Autodesk Inventor part; units mm, degrees
ref_plane "Work Plane3" through (0, 0, 250) normal (0, 0, 1) x (1, 0, 0)
ref_plane "Start Plane" through (0, 0, 0) normal (0, 0, 1) x (1, 0, 0)
ref_plane "End Plane" through (0, 0, 450) normal (0, 0, 1) x (1, 0, 0)
sketch "Sketch" plane through (0, 0, 0) normal (0, 0, 1) x (1, 0, 0)
  line L0 (-13, 15) -> (13, 15)
  line L1 (15, 13) -> (15, -13)
  line L2 (-15, 15) -> (15, -15) construction
  line L3 (15, 15) -> (-15, -15) construction
  line L4 (-5.2, 15) -> (-5.2, 14.2)
  line L5 (-5.2, 14.2) -> (-4.1, 14.2)
  line L6 (-4.1, 14.2) -> (-4.1, 12.2)
  line L7 (-4.1, 12.2) -> (-8.25, 12.2)
  line L8 (-8.25, 12.2) -> (-8.25, 10.2)
  line L9 (-8.25, 10.2) -> (-3.85, 5.8)
  line L10 (-3.85, 5.8) -> (3.85, 5.8)
  line L11 (8.25, 12.2) -> (4.1, 12.2)
  line L12 (4.1, 12.2) -> (4.1, 14.2)
  line L13 (4.1, 14.2) -> (5.2, 14.2)
  line L14 (5.2, 14.2) -> (5.2, 15)
  line L15 (8.25, 12.2) -> (8.25, 10.2)
  line L16 (8.25, 10.2) -> (3.85, 5.8)
  line L17 (-2.5, 0) -> (0, 0)
  line L18 (-5.2, -15) -> (-5.2, -14.2)
  line L19 (-5.2, -14.2) -> (-4.1, -14.2)
  line L20 (-4.1, -14.2) -> (-4.1, -12.2)
  line L21 (-4.1, -12.2) -> (-8.25, -12.2)
  line L22 (-8.25, -12.2) -> (-8.25, -10.2)
  line L23 (-8.25, -10.2) -> (-3.85, -5.8)
  line L24 (-3.85, -5.8) -> (3.85, -5.8)
  line L25 (8.25, -12.2) -> (4.1, -12.2)
  line L26 (4.1, -12.2) -> (4.1, -14.2)
  line L27 (4.1, -14.2) -> (5.2, -14.2)
  line L28 (5.2, -14.2) -> (5.2, -15)
  line L29 (8.25, -12.2) -> (8.25, -10.2)
  line L30 (8.25, -10.2) -> (3.85, -5.8)
  line L31 (15, 5.2) -> (14.2, 5.2)
  line L32 (14.2, 5.2) -> (14.2, 4.1)
  line L33 (14.2, 4.1) -> (12.2, 4.1)
  line L34 (12.2, 4.1) -> (12.2, 8.25)
  line L35 (15, -5.2) -> (14.2, -5.2)
  line L36 (14.2, -5.2) -> (14.2, -4.1)
  line L37 (14.2, -4.1) -> (12.2, -4.1)
  line L38 (12.2, -4.1) -> (12.2, -8.25)
  line L39 (12.2, -8.25) -> (10.2, -8.25)
  line L40 (10.2, -8.25) -> (5.8, -3.85)
  line L41 (5.8, -3.85) -> (5.8, 3.85)
  line L42 (5.8, 3.85) -> (10.2, 8.25)
  line L43 (10.2, 8.25) -> (12.2, 8.25)
  line L44 (-15, 5.2) -> (-14.2, 5.2)
  line L45 (-14.2, 5.2) -> (-14.2, 4.1)
  line L46 (-14.2, 4.1) -> (-12.2, 4.1)
  line L47 (-12.2, 4.1) -> (-12.2, 8.25)
  line L48 (-15, -5.2) -> (-14.2, -5.2)
  line L49 (-14.2, -5.2) -> (-14.2, -4.1)
  line L50 (-14.2, -4.1) -> (-12.2, -4.1)
  line L51 (-12.2, -4.1) -> (-12.2, -8.25)
  line L52 (-12.2, -8.25) -> (-10.2, -8.25)
  line L53 (-10.2, -8.25) -> (-5.8, -3.85)
  line L54 (-5.8, -3.85) -> (-5.8, 3.85)
  line L55 (-5.8, 3.85) -> (-10.2, 8.25)
  line L56 (-10.2, 8.25) -> (-12.2, 8.25)
  circle A0 centre (11.5, 11.5) radius 1.65
  circle A1 centre (11.5, -11.5) radius 1.65
  circle A2 centre (-11.5, 11.5) radius 1.65
  circle A3 centre (-11.5, -11.5) radius 1.65
  line L57 (-15, -13) -> (-15, -5.2)
  line L58 (-15, 5.2) -> (-15, 13)
  line L59 (13, -15) -> (5.2, -15)
  line L60 (-5.2, -15) -> (-13, -15)
  arc A4 (-13, 15) -> (-15, 13) centre (-13, 13) ccw
  arc A5 (15, 13) -> (13, 15) centre (13, 13) ccw
  arc A6 (13, -15) -> (15, -13) centre (13, -13) ccw
  arc A7 (-15, -13) -> (-13, -15) centre (-13, -13) ccw
  circle A8 centre (0, 0) radius 2.5
  point P0 (0, 0)
  point P1 (0, 5.8)
  point P2 (0, -2.5)
  point P3 (0, 2.5)
  dimension "d2" = 8.2
  dimension "d3" = 4.1
  dimension "d4" = 10.4
  dimension "d5" = 5.2
  dimension "d8" = 9.2
  dimension "d11" = 16.5
  dimension "d12" = 8.25
  dimension "d14" = 0.8
  dimension "d15" = 2
  dimension "d16" = 2
  dimension "d34" = 0.8
  dimension "d35" = 10.4
  dimension "d36" = 5.2
  dimension "d37" = 8.2
  dimension "d38" = 4.1
  dimension "d39" = 2
  dimension "d40" = 16.5
  dimension "d41" = 8.25
  dimension "d42" = 2
  dimension "d43" = 9.2
  dimension "d44" = 23
  dimension "d45" = 11.5
  dimension "d46" = 23
  dimension "d48" = 3.3
  dimension "d55" = 2
  dimension "d62" = 5
  dimension "d65" = 11.5
  dimension "d66" = 6.4
  dimension "d67" = 3.25
  dimension "d68" = 4.15
  dimension "d69" = 0.8
  dimension "d70" = 2
  dimension "d71" = 2.7577
  dimension "d72" = 5.8
  dimension "d73" = 2.7577
  dimension "d74" = 4.15
  dimension "d75" = 2
  dimension "d76" = 3.25
  dimension "d77" = 2
  dimension "d78" = 1.1
  dimension "d79" = 0.8
  dimension "d80" = 135
  dimension "d81" = 2
  dimension "d82" = 1.1
  dimension "d83" = 7.4
  dimension "d84" = 7.4
  dimension "d85" = 6.4
  dimension "d86" = 6.3
ref_plane "Work Plane3" through (0, 0, 250) normal (0, 0, 1) x (1, 0, 0)
ref_plane "Start Plane" through (0, 0, 0) normal (0, 0, 1) x (1, 0, 0)
ref_plane "End Plane" through (0, 0, 450) normal (0, 0, 1) x (1, 0, 0)
ref_plane "Start Plane1" through (0, 0, 0) normal (0, 0, 1) x (1, 0, 0)
ref_plane "End Plane1" through (0, 0, 450) normal (0, 0, 1) x (1, 0, 0)
ref_plane "Start Plane2" through (0, 0, 15) normal (0, 0, 1) x (1, 0, 0)
ref_plane "End Plane2" through (0, 0, 435) normal (0, 0, 1) x (1, 0, 0)
extrude "Body" add sketch "Sketch" along normal up to surface (420 mm away) from surface at 15 contours L0 L4 L5 L6 L7 L8 L9 L10 L16 L15 L11 L12 L13 L14 A5 L1 L31 L32 L33 L34 L43 L42 L41 L40 L39 L38 L37 L36 L35 A6 L59 L28 L27 L26 L25 L29 L30 L24 L23 L22 L21 L20 L19 L18 L60 A7 L57 L48 L49 L50 L51 L52 L53 L54 L55 L56 L47 L46 L45 L44 L58 A4
sketch "Sketch7" plane through (0, 0, 0) normal (0, 0, 1) x (1, 0, 0)
  line L0 (0, 0) -> (10, 0)
ref_plane "Work Plane10" through (0, 0, 0) normal (0, -1, 0) x (1, 0, 0)
sketch "Sketch8" plane through (0, 0, 0) normal (0, -1, 0) x (1, 0, 0)
  line L0 (-2, 15) -> (12, 15)
  line L1 (-2, 435) -> (12, 435)
  dimension "d100" = 420
equation "\"d38\" = 0.5 * d37"
equation "\"d41\" = 0.5 * d40"
equation "\"d45\" = 0.5 * d44"
equation "\"G_OFFSET_START\" = 0"
equation "\"G_OFFSET_END\" = 0"
equation "\"G_L\" = 500"
equation "\"G_OFFSET_START1\" = 0"
equation "\"G_OFFSET_END1\" = 0"
equation "\"G_OFFSET_START2\" = -15"
equation "\"G_OFFSET_END2\" = -15"
equation "\"d95\" = -G_OFFSET_START2"
equation "\"d96\" = Length + G_OFFSET_END2"
properties part number "420 mm" material "Aluminum 6061"
Work out the finished part from the listing and answer in its coordinate system (mm). A direction names the side the tool comes from. Give positions to 0.01 mm unless a question says otherwise; leave off trailing zeros. Use a Markdown table: item, result. Add a question column.
1. Section A-A on z = 279 is taken. State how many separate pieces and enclosed holes the cut face has, and give its area (3 significant figures).
2. For faces 5 (the flat face through (5.8, 0, 222)), 6 (the flat face through (15, 9, 222)), 7 (the flat face through (-5.8, 0, 222)), determine the directions among +Z, -Z, +X, -X, +Y, -Y from which every point of the face is accessible in a straight line to the end or side of a thin tool.
3. Find the intervals of material crossed by probe 1 along Y at (x, z) = (11.5, 242); probe 2 along X at (y, z) = (-11.25, 88); probe 3 along Y at (x, z) = (-5.25, 263), in increasing order.
4. Determine the mould class of faces 1 (the flat face through (0, 5.8, 222)), 2 (the flat face through (0, -5.8, 222)), 3 (the flat face through (0, 4, 435)), 4 (the flat face through (-15, -9, 222)) for opening direction X: released by +X, released by -X, zero draft, split by the parting line, or undercut.
5. Flat-ended cylindrical pins translate along their axes: pin 1 Ø6 at (x, z) = (-1.5, 153.5) entering from +Y; pin 2 Ø8.5 at (x, z) = (-1.5, 212) entering from -Y; pin 3 Ø8.5 at (y, z) = (0.5, 255) entering from +X; pin 4 Ø0.6 at (x, z) = (-4.5, 196) entering from -Y. Find the tip coordinate at first contact, or state that the pin passes through.
Results below:
| question | item | result |
|---|---|---|
| 1 | separate pieces | 1 |
| 1 | enclosed holes | 5 |
| 1 | area | 399 mm^2 |
| 2 | face 5 | +Z, -Z, +X |
| 2 | face 6 | +Z, -Z, +X, +Y, -Y |
| 2 | face 7 | +Z, -Z, -X |
| 3 | probe 1 | y = -15 to -13.15, -9.85 to -8.25, 8.25 to 9.85, 13.15 to 15 |
| 3 | probe 2 | x = -15 to -13.13, -9.87 to -8.25, 8.25 to 9.87, 13.13 to 15 |
| 3 | probe 3 | y = -15 to -12.2, -7.2 to 7.2, 12.2 to 15 |
| 4 | face 1 | undercut |
| 4 | face 2 | undercut |
| 4 | face 3 | zero draft |
| 4 | face 4 | released by -X |
| 5 | pin 1 | stops at y = 14.2 |
| 5 | pin 2 | stops at y = -15 |
| 5 | pin 3 | stops at x = 14.2 |
| 5 | pin 4 | stops at y = -14.2 |
